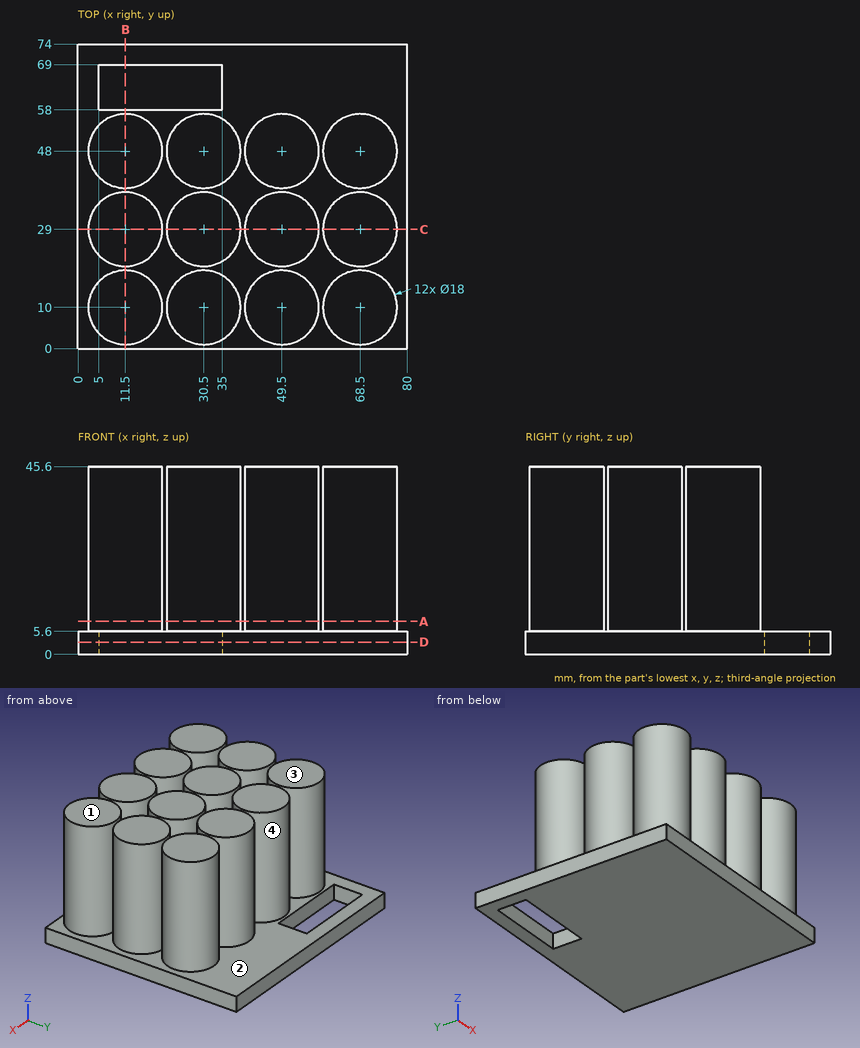
Drawing for the job (mm, zero at the part's lowest x, y, z). A direction names the side the tool comes from. Give positions to 0.01 mm unless a question says otherwise; leave off trailing zeros. Write each loop counter-clockwise with the first axis right and the second up, starting at its lowest first coordinate (ties: lowest second). Pieces come first, ordered by that corner, then holes. Notation, with made-up numbers: (65, 39.5) - (123, 39.5) arc R16 ccw to (123, 62.5) - close; hole circle Ø8 at (22, 79). An arc over 180 degrees is marked (long way). Answer as CSV lines item,"result".
Q1. Band-saw the part on D-D (z = 3). Give the cut face in (x, y).
Result set:
outline,"(0, 0) - (80, 0) - (80, 74) - (0, 74) - close; hole (5, 58) - (35, 58) - (35, 69) - (5, 69) - close"
Q2. Pull direction Y, two halves, no side cores. Call the marked faces 1 and 2: released by +Y, released by -Y, zero draft, split by the parting line, or undercut.
Result set:
face 1,"zero draft"
face 2,"undercut"
Q3. Drill centre lines: line 1 (Y direction, x = 30.5, z = 6); line 2 (Y direction, x = 29, z = 31.5); line 3 (X direction, y = 4, z = 24). Where is each one in solid material? Low to high. Write a range as from..to.
Result set:
line 1,"1..19, 20..38, 39..57"
line 2,"1.13..18.87, 20.13..37.87, 39.13..56.87"
line 3,"4.79..18.21, 23.79..37.21, 42.79..56.21, 61.79..75.21"
Q4. Band-saw the part on C-C (y = 29). Give the cut face in (x, z).
Result set:
outline,"(0, 0) - (80, 0) - (80, 5.6) - (77.5, 5.6) - (77.5, 45.6) - (59.5, 45.6) - (59.5, 5.6) - (58.5, 5.6) - (58.5, 45.6) - (40.5, 45.6) - (40.5, 5.6) - (39.5, 5.6) - (39.5, 45.6) - (21.5, 45.6) - (21.5, 5.6) - (20.5, 5.6) - (20.5, 45.6) - (2.5, 45.6) - (2.5, 5.6) - (0, 5.6) - close"
Q5. Band-saw the part on A-A (z = 8). State how many separate pieces and enclosed holes the cut face has, and give its area (3 significant figures).
Result set:
separate pieces,"12"
enclosed holes,"0"
area,"3,050 mm²"
Q6. Flat gauge pins, fed straight in: pin 1 Ø1 at (x, z) = (19, 24) entering from -Y; pin 2 Ø8 at (x, z) = (69.5, 40) entering from +Y; pin 3 Ø1.5 at (y, z) = (30, 37.5) entering from -X. Where does each tip first touch, or does it go through?
Result set:
pin 1,"y = 4.34"
pin 2,"y = 57"
pin 3,"x = 2.5"
Q7. 3-axis set-ups, long thin cutter, end or side, ignore diameter. For the marked faces 3 and 4: which of +Z, -Z, +X, -X, +Y, -Y reach the whole face in a straight line?
Result set:
face 3,"+Z, +X, -X, +Y, -Y"
face 4,"+Z"
Q8. Band-saw the part on B-B (x = 11.5). Give the cut face in (y, z), and give its area (3 significant figures).
Result set:
outline,"(0, 0) - (58, 0) - (58, 5.6) - (57, 5.6) - (57, 45.6) - (39, 45.6) - (39, 5.6) - (38, 5.6) - (38, 45.6) - (20, 45.6) - (20, 5.6) - (19, 5.6) - (19, 45.6) - (1, 45.6) - (1, 5.6) - (0, 5.6) - close; (69, 0) - (74, 0) - (74, 5.6) - (69, 5.6) - close"
area,"2,510 mm²"
